Drawing for the job (mm, zero at the part's lowest x, y, z). A direction names the side the tool comes from. Coordinates: 2 decimals unless noted, no trailing zeros. Write each loop counter-clockwise with the first axis right and the second up, starting at its lowest first coordinate (ties: lowest second). Pieces come first, ordered by that corner, then holes. Notation, with made-up numbers: (53, 48) -> (109, 48) arc R19 cw to (109, 63) -> close; hole circle Ø11 at (8.25, 10.5). An arc over 180 degrees is marked (long way). Answer as CSV lines item,"result".
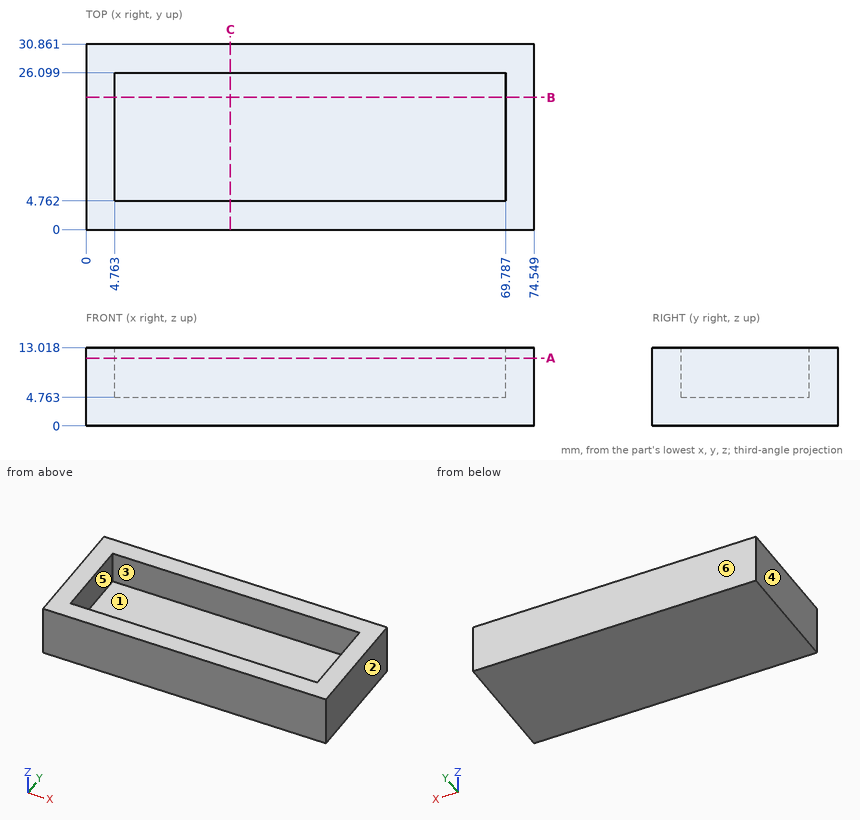
Item 1: Saw through at C-C on x = 24. Give the cut face in (y, z).
Answer below:
outline,"(0, 0) -> (30.86, 0) -> (30.86, 13.02) -> (26.1, 13.02) -> (26.1, 4.76) -> (4.76, 4.76) -> (4.76, 13.02) -> (0, 13.02) -> close"
Item 2: Saw through at B-B on y = 22. Give the cut face in (x, z).
Answer below:
outline,"(0, 0) -> (74.55, 0) -> (74.55, 13.02) -> (69.79, 13.02) -> (69.79, 4.76) -> (4.76, 4.76) -> (4.76, 13.02) -> (0, 13.02) -> close"
Item 3: Wall check: line 1 (Y direction, x = 58, z = 8); line 2 (X direction, y = 13.5, z = 9.75); line 3 (Z direction, x = 62.5, y = 7.5). Give the ranges that are in metal, low to high. Write a range as from..to.
Answer below:
line 1,"y = 0..4.76, 26.1..30.86"
line 2,"x = 0..4.76, 69.79..74.55"
line 3,"z = 0..4.76"
Item 4: 3-axis set-ups, long thin cutter, end or side, ignore diameter. For the marked faces 1 and 2: which of +Z, -Z, +X, -X, +Y, -Y reach the whole face in a straight line?
Answer below:
face 1,"+Z"
face 2,"+Z, -Z, +X, +Y, -Y"
Item 5: Saw through at A-A on z = 11.25. Give the cut face in (x, y).
Answer below:
outline,"(0, 0) -> (74.55, 0) -> (74.55, 30.86) -> (0, 30.86) -> close; hole (4.76, 4.76) -> (69.79, 4.76) -> (69.79, 26.1) -> (4.76, 26.1) -> close"
Item 6: Two-plate mould, pull along X, no slides. Class the marked faces 3, 4, 5 and 6: pulls with the +X half, pulls with the -X half, needs draft (parallel to the pull), parting line crosses it, or undercut.
Answer below:
face 3,"undercut"
face 4,"pulls with the -X half"
face 5,"undercut"
face 6,"needs draft"
Item 7: Flat gauge pin, fed straight in: pin 1 (12 mm diameter, centred on x = 38, y = 19.5, fed in from +Z). Where does the tip first touch, or does it go through?
Answer below:
pin 1,"stops at z = 4.76"
